Autodesk Inventor part; units mm, degrees
ref_plane "YZ Plane" through (0, 0, 0) normal (1, 0, 0) x (0, 1, 0)
ref_plane "XZ Plane" through (0, 0, 0) normal (0, 1, 0) x (-1, 0, 0)
ref_plane "XY Plane" through (0, 0, 0) normal (0, 0, 1) x (1, 0, 0)
sketch "Sketch9" plane through (0, 0, 0) normal (0, 0, 1) x (1, 0, 0)
  line L0 (0, 0) -> (130, 0)
  line L1 (130, 0) -> (130, 130)
  line L2 (130, 130) -> (0, 130)
  line L3 (0, 130) -> (0, 0)
  dimension "d32" = 130
  dimension "d33" = 130
extrude "Extrusion9" add sketch "Sketch9" along normal blind 30
sketch "Sketch10" plane through (0, 0, 30) normal (0, 0, 1) x (1, 0, 0)
  line L0 (0, 130) -> (0, 0)
  line L1 (130, 0) -> (130, 130)
  line L2 (0, 130) -> (130, 0) construction
  circle A0 centre (65, 65) radius 23.8125
  dimension "d36" = 47.625
extrude "Extrusion10" cut sketch "Sketch10" against normal blind 40
sketch "Sketch11" plane through (0, 0, 0) normal (-1, 0, 0) x (0, 0, 1)
  point P0 (0, 0)
sketch "Sketch12" plane through (0, 0, 0) normal (0, -1, 0) x (1, 0, 0)
  line L0 (130, 0) -> (130, 30)
  line L1 (0, 0) -> (130, 0)
  line L2 (130, 0) -> (130, 30)
  line L3 (130, 30) -> (0, 30)
  line L4 (0, 30) -> (0, 0)
extrude "Extrusion11" add sketch "Sketch12" along normal blind 40
sketch "Sketch13" plane through (0, -40, 0) normal (0, -1, 0) x (1, 0, 0)
  line L0 (130, 30) -> (0, 30)
  line L1 (0, 0) -> (130, 0)
  line L2 (130, 0) -> (130, 30)
  line L3 (130, 30) -> (0, 30)
  line L4 (0, 30) -> (0, 0)
  point P0 (0, 30)
extrude "Extrusion12" cut sketch "Sketch13" against normal blind 20
sketch "Sketch15" plane through (0, -20, 0) normal (0, -1, 0) x (1, 0, 0)
  line L0 (130, 30) -> (0, 30)
  line L1 (130, 30) -> (0, 30)
  line L2 (0, 30) -> (0, 0)
  line L3 (0, 0) -> (130, 0)
  line L4 (130, 0) -> (130, 30)
  point P0 (0, 30)
extrude "Extrusion14" add sketch "Sketch15" along normal blind 40
sketch "Sketch16" plane through (0, -60, 0) normal (0, -1, 0) x (1, 0, 0)
  line L0 (130, 30) -> (0, 30)
  line L1 (130, 30) -> (0, 30)
  line L2 (0, 30) -> (0, 0)
  line L3 (0, 0) -> (130, 0)
  line L4 (130, 0) -> (130, 30)
extrude "Extrusion15" cut sketch "Sketch16" against normal blind 15
sketch "Sketch17" plane through (0, -45, 0) normal (0, -1, 0) x (1, 0, 0)
  line L0 (130, 30) -> (0, 30)
  line L1 (130, 30) -> (0, 30)
  line L2 (0, 30) -> (0, 0)
  line L3 (0, 0) -> (130, 0)
  line L4 (130, 0) -> (130, 30)
extrude "Extrusion16" cut sketch "Sketch17" against normal blind 10
sketch "Sketch19" plane through (0, -35, 0) normal (0, -1, 0) x (1, 0, 0)
  circle A0 centre (25, 15) radius 10.682
  line L0 (0, 30) -> (130, 30)
  line L1 (0, 0) -> (0, 30)
  dimension "d64" = 21.364
  dimension "d65" = 15
  dimension "d66" = 25
extrude "Extrusion18" add sketch "Sketch19" along normal blind 15
sketch "Sketch20" plane through (0, -35, 0) normal (0, -1, 0) x (1, 0, 0)
  line L0 (0, 0) -> (0, 30)
  line L1 (0, 30) -> (130, 30)
  line L2 (0, 0) -> (130, 0)
  line L3 (130, 0) -> (130, 30)
  line L4 (130, 30) -> (0, 30)
  line L5 (0, 30) -> (0, 0)
extrude "Extrusion19" add sketch "Sketch20" along normal blind 25
sketch "Sketch21" plane through (0, -60, 0) normal (0, -1, 0) x (1, 0, 0)
  circle A0 centre (15, 15) radius 10.682
  line L0 (130, 30) -> (0, 30)
  line L1 (0, 30) -> (0, 0)
  dimension "d71" = 21.364
  dimension "d72" = 15
  dimension "d73" = 15
extrude "Extrusion20" add sketch "Sketch21" along normal blind 25
properties part number "Spring connection"
Can you work these out from the model? Positions are in its coordinate system, mm. A direction names the side the tool comes from. Coordinates: 2 decimals unless noted, no trailing zeros. Write each loop counter-clockwise with the first axis right and the second up, starting at its lowest first coordinate (ties: lowest second). Pieces come first, ordered by that corner, then holes. Notation, with made-up numbers: (56, 16.5) -> (88, 16.5) arc R17 cw to (88, 33.5) -> close; hole circle Ø8 at (75.25, -37). An arc over 180 degrees is marked (long way). Write item = value, one per line.
(1) On a 3-axis mill with a long thin cutter (end or side, diameter ignored), from which of +Z, -Z, +X, -X, +Y, -Y can I reach the whole of each face in a straight line? I mean faces 4 (the face through (24.87, -72.32, 19.09)), 5 (the face through (64, 36, 0)). Say none if no direction works.
Verdict:
face_4 = -Y
face_5 = -Z, +X, -X, +Y, -Y
(2) Imagine slicing it at A-A (z = 15). Please give me the cut outline in (x, y) (1 decimal).
Verdict:
outline = (0, -60) -> (4.3, -60) -> (4.3, -85) -> (25.7, -85) -> (25.7, -60) -> (130, -60) -> (130, 130) -> (0, 130) -> close; hole circle Ø47.6 at (65, 65)
(3) Imagine slicing it at D-D (x = 95). Please give me the cut outline in (y, z), and give its area (3 significant figures).
Verdict:
outline = (-60, 0) -> (130, 0) -> (130, 30) -> (-60, 30) -> close
area = 5,700 mm^2
(4) If I drill on probe 1 along Y at (x, z) = (65, 15.5); probe 2 along Y at (x, z) = (32, 19.75); probe 3 along X at (y, z) = (46.5, 2.75), over which ranges is the centre line in solid material (lowest first)?
Verdict:
probe_1 = -60 to 41.19, 88.81 to 130
probe_2 = -60 to 130
probe_3 = 0 to 50.01, 79.99 to 130
(5) Imagine slicing it at B-B (y = 65). Please give me the cut outline in (x, z), and give its area (3 significant figures).
Verdict:
outline = (0, 0) -> (41.19, 0) -> (41.19, 30) -> (0, 30) -> close; (88.81, 0) -> (130, 0) -> (130, 30) -> (88.81, 30) -> close
area = 2,470 mm^2
(6) Imagine slicing it at C-C (x = 62). Please give me the cut outline in (y, z), and give its area (3 significant figures).
Verdict:
outline = (-60, 0) -> (41.38, 0) -> (41.38, 30) -> (-60, 30) -> close; (88.62, 0) -> (130, 0) -> (130, 30) -> (88.62, 30) -> close
area = 4,280 mm^2
(7) Thinking about a two-plate mould opening in X: for faces 1 (the face through (130, 36, 15)), 2 (the face through (64, 36, 30)), 3 (the face through (47.449, 81.094, 15.21)), which applies, +X half, -X half, draft (parallel to the pull), parting line (faces both ways), or undercut?
Verdict:
face_1 = +X half
face_2 = draft
face_3 = undercut
